```python
from build123d import *

# Parameters (mm, degrees)
F0_W     = 12.7
F0_H     = 12.7
F1_DEPTH = 12.7
F2_W     = 6.35
F2_H     = 6.35
F3_DEPTH = 12.7
F5_DEPTH = 6.35


with BuildPart() as f1:
    # F0 (on Front) → F1 (new body)
    with BuildSketch(Plane.XZ):
        with Locations((-18.813286, 29.219552)):
            Rectangle(F0_W, F0_H)
        Polygon((-12.463286, 22.869552), (-25.163286, 22.869552), (-25.163286, 16.519552), (4.999214, 16.519552), (4.999214, 22.869552), align=None)
    extrude(amount=F1_DEPTH)

    # F2 (on face) → F3 (join)
    with BuildSketch(Plane.XY.offset(22.869552)):
        with Locations((1.824214, -3.175)):
            Rectangle(F2_W, F2_H)
    extrude(amount=F3_DEPTH)

    # F4 (on face) → F5 (join)
    with BuildSketch(Plane(origin=(0, 0, 0), x_dir=(-1, 0, 0), z_dir=(0, 1, 0))):
        Polygon((12.463286, 22.869552), (1.350786, 35.569552), (1.350786, 22.869552), align=None)
    extrude(amount=-F5_DEPTH)


solid = f1.part
```
The listing builds one solid part. Answer for the finished solid, in the listing's coordinates (mm). A direction names the side the tool comes from. Round coordinates to 2 decimals unless told otherwise and drop trailing zeros. Loops run counter-clockwise (first coordinate to the right, second up) from the corner with the lowest first, then second, coordinate; pieces in that order, holes last. Notation, with made-up numbers: (62.5, -36.75) - (99.5, -36.75) arc R34 ccw to (99.5, 1.25) - close; hole circle Ø8 at (-25.75, 45.5). An arc over 180 degrees is marked (long way). Return JSON: item names as keys, results as strings. Group by question number.
1. Each of these flat-tipped pins is pushed along its axis until it touches: P1, Ø1.9, axis at x = -8, y = -9, coming from the +Z side; P2, Ø4, axis at x = -9.5, y = -6.5, coming from the +Z side; P3, Ø6, axis at x = -18.5, z = 30, coming from the +Y side; P4, Ø4, axis at x = -7.5, z = 30, coming from the -Y side. Where does it stop, or does it pass through?
2. Which of the six approach directions +Z, -Z, +X, -X, +Y, -Y give full straight-line access (tool end or side, diameter ignored) to faces 1 (the flat face through (-4, -9, 22.87)), 2 (the flat face through (-12.463, -6, 29)), 3 (the flat face through (-19, -6, 35.57))?
3. The part is cut by section C-C on z = 28.5. Determine the outline of the cut face in (x, y), then the cut area to 3 significant figures.
4. The part is cut by section D-D on x = -4.5. Determine the outline of the cut face in (y, z), then the cut area to 3 significant figures.
5. The part is cut by section A-A on z = 26.5. Determine the outline of the cut face in (x, y).
6. The mould has two halves that part along X. Classify faces 4 (the flat face through (-6.985, -3.131, 29.131)), 5 (the flat face through (-25.163, -6, 26)), 6 (the flat face through (-10, -6, 16.52)), 7 (the flat face through (4.999, -5, 24)): pulls with the +X half, pulls with the -X half, needs draft (parallel to the pull), parting line crosses it, or undercut.
7. The part is cut by section B-B on y = -8. Determine the outline of the cut face in (x, z), then the cut area to 3 significant figures.
8. Consider probe 1 along X at (y, z) = (-9.75, 28.75); probe 2 along Y at (x, z) = (-2, 32); probe 3 along X at (y, z) = (-1.5, 34). Determine where each line is inside the solid, lowest interval first.
Resolved:
{
 "1": {"P1": "stops at z = 22.87", "P2": "stops at z = 28.54", "P3": "stops at y = 0", "P4": "stops at y = -6.35"},
 "2": {"face 1": "+Z, +X, -Y", "face 2": "+Z, +Y, -Y", "face 3": "+Z, +X, -X, +Y, -Y"},
 "3": {"outline": "(-25.16, -12.7) - (-12.46, -12.7) - (-12.46, 0) - (-25.16, 0) - close; (-7.54, -6.35) - (5, -6.35) - (5, 0) - (-7.54, 0) - close", "area": "241 mm²"},
 "4": {"outline": "(-12.7, 16.52) - (0, 16.52) - (0, 31.97) - (-6.35, 31.97) - (-6.35, 22.87) - (-12.7, 22.87) - close", "area": "138 mm²"},
 "5": {"outline": "(-25.16, -12.7) - (-12.46, -12.7) - (-12.46, 0) - (-25.16, 0) - close; (-9.29, -6.35) - (5, -6.35) - (5, 0) - (-9.29, 0) - close"},
 "6": {"face 4": "undercut", "face 5": "pulls with the -X half", "face 6": "needs draft", "face 7": "pulls with the +X half"},
 "7": {"outline": "(-25.16, 16.52) - (5, 16.52) - (5, 22.87) - (-12.46, 22.87) - (-12.46, 35.57) - (-25.16, 35.57) - close", "area": "353 mm²"},
 "8": {"probe 1": "x = -25.16 to -12.46", "probe 2": "y = -6.35 to 0", "probe 3": "x = -25.16 to -12.46, -2.72 to 5"}
}
